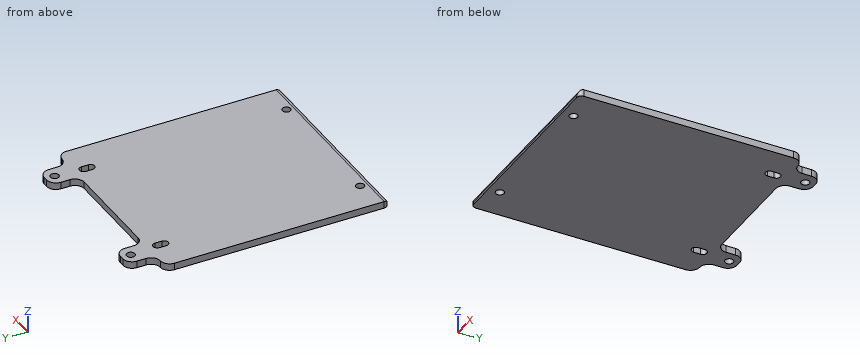
```python
from build123d import *

# Parameters (mm, degrees)
SKETCH1_R           = 1.8
BOSS_EXTRUDE1_DEPTH = 3
FILLET1_R           = 4
FILLET2_R           = 2


with BuildPart() as part:
    # Sketch1 → Boss-Extrude1 (new body)
    with BuildSketch(Plane.XY):
        Polygon((-88, 0), (0, 0), (0, 97), (-8, 97), (-8, 109), (-18, 109), (-18, 97), (-70, 97), (-70, 109), (-80, 109), (-80, 97), (-88, 97), align=None)
        with Locations((-74, 5)):
            Circle(SKETCH1_R, mode=Mode.SUBTRACT)
        with Locations((-14, 5)):
            Circle(SKETCH1_R, mode=Mode.SUBTRACT)
        with BuildLine():
            ThreePointArc((-75.8, 93), (-74, 94.8), (-72.2, 93))
            Line((-72.2, 93), (-72.2, 90))
            ThreePointArc((-72.2, 90), (-74, 88.2), (-75.8, 90))
            Line((-75.8, 90), (-75.8, 93))
        make_face(mode=Mode.SUBTRACT)
        with BuildLine():
            ThreePointArc((-12.2, 90), (-14, 88.2), (-15.8, 90))
            Line((-15.8, 90), (-15.8, 93))
            ThreePointArc((-15.8, 93), (-14, 94.8), (-12.2, 93))
            Line((-12.2, 93), (-12.2, 90))
        make_face(mode=Mode.SUBTRACT)
        with Locations((-13, 105)):
            Circle(SKETCH1_R, mode=Mode.SUBTRACT)
        with Locations((-75, 105)):
            Circle(SKETCH1_R, mode=Mode.SUBTRACT)
    extrude(amount=BOSS_EXTRUDE1_DEPTH)

    # Fillet1
    fillet1_edges = [part.edges().sort_by_distance(p)[0] for p in [
        (-70, 109, 1.5),
        (-70, 97, 1.5),
        (-18, 97, 1.5),
        (-18, 109, 1.5),
        (-8, 109, 1.5),
        (-8, 97, 1.5),
        (0, 97, 1.5),
        (-88, 97, 1.5),
        (-80, 97, 1.5),
        (-80, 109, 1.5),
    ]]
    fillet(fillet1_edges, radius=FILLET1_R - 0.0001)  # a hair under: the kernel refuses the full size

    # Fillet2
    fillet2_edges = [part.edges().sort_by_distance(p)[0] for p in [
        (-44, 0, 3),
        (0, 0, 1.5),
        (-88, 0, 1.5),
    ]]
    fillet(fillet2_edges, radius=FILLET2_R)


solid = part.part
```
The model under review builds one solid part; all positions refer to its coordinate system, in mm. Give positions to 0.01 mm unless a question says otherwise; leave off trailing zeros. Write each loop counter-clockwise with the first axis right and the second up, starting at its lowest first coordinate (ties: lowest second). Pieces come first, ordered by that corner, then holes. Notation, with made-up numbers: M 13,-32.75 L 65,-32.75 A22 cw 65,-2.75 Z; hole C 81,88 d1. An arc over 180 degrees is marked long. Write each question's results on one line, items separated by ' | '. Start each with the question number.
1. For probe 1 along X at (y, z) = (93, 2.1); probe 2 along Y at (x, z) = (-74, 2.15); probe 3 along Y at (x, z) = (-75, 0.9), list the stretches that pass through material, from the lowest coordinate up. Write a range as [from, to].
2. We need section C-C (z = 1.8). Count the separate pieces of the cut face and the enclosed holes in it, and give its area (3 significant figures).
3. We need section D-D (x = -81.5). Write out the cut boundary in (y, z), and give its area (3 significant figures).
4. We need section A-A (y = 5). Write out the cut boundary in (x, z).
5. We need section B-B (x = -39). Write out the cut boundary in (y, z).
6. Insertion check: pin 1 Ø1.5 at (x, z) = (-43.5, 1) entering from +Y; pin 2 Ø0.9 at (y, z) = (102, 1) entering from +X. Each pin has a flat end and moves straight along its axis. Give the tip position at first contact, or say it passes through.
Results found:
1) probe 1: x = [-88, -75.8], [-72.2, -15.8], [-12.2, 0] | probe 2: y = [0.36, 3.2], [6.8, 88.2], [94.8, 103.5], [106.5, 109] | probe 3: y = [0, 3.5], [6.5, 88.5], [94.5, 103.2], [106.8, 109]
2) separate pieces: 1 | enclosed holes: 6 | area: 8,670 mm^2
3) outline: M 0,0 L 97.88,0 L 97.88,3 L 2,3 A2 ccw 0,1 Z | area: 293 mm^2
4) outline: M -88,0 L -75.8,0 L -75.8,3 L -88,3 Z; M -72.2,0 L -15.8,0 L -15.8,3 L -72.2,3 Z; M -12.2,0 L 0,0 L 0,3 L -12.2,3 Z
5) outline: M 0,0 L 97,0 L 97,3 L 2,3 A2 ccw 0,1 Z
6) pin 1: stops at y = 97 | pin 2: stops at x = -8
